Read the model definition and answer for the solid it produces. Units are mm, in the model's axes. Coordinates: 2 decimals unless noted, no trailing zeros. Write each loop counter-clockwise with the first axis right and the second up, starting at its lowest first coordinate (ties: lowest second). Pieces come first, ordered by that corner, then holes.
(1) Section A-A on y = 200 is taken. Write down the section's boundary in (x, z).
(2) Given pin 1 (1 mm diameter, centred on x = -6, z = -1.5, fed in from -Y); pin 2 (4 mm diameter, centred on x = 0, z = -0.5, fed in from -Y); pin 3 (10 mm diameter, centred on y = 219.5, z = 6, fed in from -X), each flat-ended and moving along its own axis, determine where each tip first touches the part or whether it passes through.
(3) Find the intervals of material crossed by probe 1 along X at (y, z) = (38, 0); probe 2 along Y at (x, z) = (-12.5, 7.5); probe 3 along Z at (x, y) = (0.5, 278), in increasing order.
(4) The mould has two halves that part along Y. Classify faces 1 (the cylindrical face through (4.88, 322.16, 1.08)), 2 (the conical face through (2.172, 50.809, 2.833)), 3 (the cylindrical face through (-0.9, 183.02, -2.86)), 4 (the flat face through (0, 335.233, 0)): +Y half, -Y half, draft (parallel to the pull), parting line (faces both ways), or undercut.
from build123d import *


with BuildPart() as part:
    # Sketch1 → Revolve2 (revolve)
    with BuildSketch(Plane.XY, mode=Mode.PRIVATE) as revolve2_sk:
        with BuildLine():
            Line((-5, 327.232699925), (-5, 317.232699925))
            add(Edge.make_bspline(
                [(-5, 317.232699925), (-3.994069006, 317.33794331), (-3, 317.520687178)],
                knots=[0, 0, 0, 1, 1, 1], degree=2))
            Line((-3, 317.520687178), (-3, 52.232699925))
            Line((-3, 52.232699925), (-5, 47.232699925))
            Line((-5, 47.232699925), (-5, 35.232699925))
            Line((-5, 35.232699925), (-4, 35.232699925))
            Line((-4, 35.232699925), (-4, 46.232699925))
            Line((-4, 46.232699925), (0, 46.232699925))
            Line((0, 46.232699925), (0, 335.232699925))
            Line((0, 335.232699925), (-25, 335.232699925))
            ThreePointArc((-25, 335.232699925), (-26.656854249, 331.232699925), (-25, 327.232699925))
            Line((-25, 327.232699925), (-5, 327.232699925))
        make_face()
    revolve(revolve2_sk.sketch.rotate(Axis((0, 0, 0), (0, 1, 0)), 270), axis=Axis((0, 0, 0), (0, 1, 0)))


solid = part.part
Response:
1. outline: circle Ø6 at (0, 0)
2. pin 1: stops at y = 327.23
2. pin 2: stops at y = 46.23
2. pin 3: stops at x = -2.83
3. probe 1: x = -5 to -4, 4 to 5
3. probe 2: y = 327.23 to 335.23
3. probe 3: z = -2.96 to 2.96
4. face 1: draft
4. face 2: undercut
4. face 3: undercut
4. face 4: +Y half
